from build123d import *

# Parameters (mm, degrees)
SKETCH1_R           = 4.9022
SKETCH1_W           = 40
SKETCH1_H           = 2.6
SKETCH1_W_2         = 80
BOSS_EXTRUDE4_DEPTH = 10


with BuildPart() as part:
    # Sketch1 → Boss-Extrude4 (new body)
    with BuildSketch(Plane(origin=(0, 0, 0), x_dir=(1, 0, 0), z_dir=(0, 1, 0))):
        Polygon((-60.000001624, 254.034119381), (60.000003913, 254.034119381), (250.000001144, -75.055535655), (189.999998376, -178.978582511), (-190.000001624, -178.978582511), (-250.000001624, -75.055534057), align=None)
        with Locations(Location((-200.000000812, -115.470053369, 0), (0, 0, 270))):
            Circle(SKETCH1_R, mode=Mode.SUBTRACT)
        with Locations(Location((199.99999988, -115.470053769, 0), (0, 0, 270))):
            Circle(SKETCH1_R, mode=Mode.SUBTRACT)
        with Locations(Location((5.72e-07, 230.940108145, 0), (0, 0, 270))):
            Circle(SKETCH1_R, mode=Mode.SUBTRACT)
        Polygon((-191.125833025, -87.252540378), (-188.874166975, -85.952540378), (-168.874166975, -120.59355653), (-171.125833025, -121.89355653), align=None, mode=Mode.SUBTRACT)
        with Locations((0, 207.846096908)):
            Rectangle(SKETCH1_W, SKETCH1_H, mode=Mode.SUBTRACT)
        Polygon((188.874166975, -85.952540378), (191.125833025, -87.252540378), (171.125833025, -121.89355653), (168.874166975, -120.59355653), align=None, mode=Mode.SUBTRACT)
        Polygon((148.874166975, -16.670508076), (151.125833025, -17.970508076), (131.125833025, -52.611524227), (128.874166975, -51.311524227), align=None, mode=Mode.SUBTRACT)
        Polygon((-51.125833025, 52.611524227), (-48.874166975, 51.311524227), (-68.874166975, 16.670508076), (-71.125833025, 17.970508076), align=None, mode=Mode.SUBTRACT)
        Polygon((-11.125833025, 121.89355653), (-8.874166975, 120.59355653), (-28.874166975, 85.952540378), (-31.125833025, 87.252540378), align=None, mode=Mode.SUBTRACT)
        Polygon((28.874166975, 52.611524227), (31.125833025, 51.311524227), (11.125833025, 16.670508076), (8.874166975, 17.970508076), align=None, mode=Mode.SUBTRACT)
        Polygon((-61.125833025, 173.855080757), (-58.874166975, 172.555080757), (-98.874166975, 103.273048454), (-101.125833025, 104.573048454), align=None, mode=Mode.SUBTRACT)
        Polygon((-141.125833025, 35.291016151), (-138.874166975, 33.991016151), (-178.874166975, -35.291016151), (-181.125833025, -33.991016151), align=None, mode=Mode.SUBTRACT)
        with Locations((40, 138.564064606)):
            Rectangle(SKETCH1_W, SKETCH1_H, mode=Mode.SUBTRACT)
        with Locations((80, -69.282032303)):
            Rectangle(SKETCH1_W, SKETCH1_H, mode=Mode.SUBTRACT)
        with Locations((-80, -138.564064606)):
            Rectangle(SKETCH1_W_2, SKETCH1_H, mode=Mode.SUBTRACT)
        with Locations((80, -138.564064606)):
            Rectangle(SKETCH1_W_2, SKETCH1_H, mode=Mode.SUBTRACT)
        Polygon((-111.125833025, -87.252540378), (-108.874166975, -85.952540378), (-88.874166975, -120.59355653), (-91.125833025, -121.89355653), align=None, mode=Mode.SUBTRACT)
        Polygon((-71.125833025, -17.970508076), (-68.874166975, -16.670508076), (-48.874166975, -51.311524227), (-51.125833025, -52.611524227), align=None, mode=Mode.SUBTRACT)
        Polygon((8.874166975, -17.970508076), (11.125833025, -16.670508076), (31.125833025, -51.311524227), (28.874166975, -52.611524227), align=None, mode=Mode.SUBTRACT)
        Polygon((48.874166975, 51.311524227), (51.125833025, 52.611524227), (71.125833025, 17.970508076), (68.874166975, 16.670508076), align=None, mode=Mode.SUBTRACT)
        Polygon((58.863601684, 172.573380377), (61.115267734, 173.873380377), (101.115267734, 104.591348074), (98.863601684, 103.291348074), align=None, mode=Mode.SUBTRACT)
        Polygon((138.874166975, 33.991016151), (141.125833025, 35.291016151), (181.125833025, -33.991016151), (178.874166975, -35.291016151), align=None, mode=Mode.SUBTRACT)
    extrude(amount=BOSS_EXTRUDE4_DEPTH)


solid = part.part
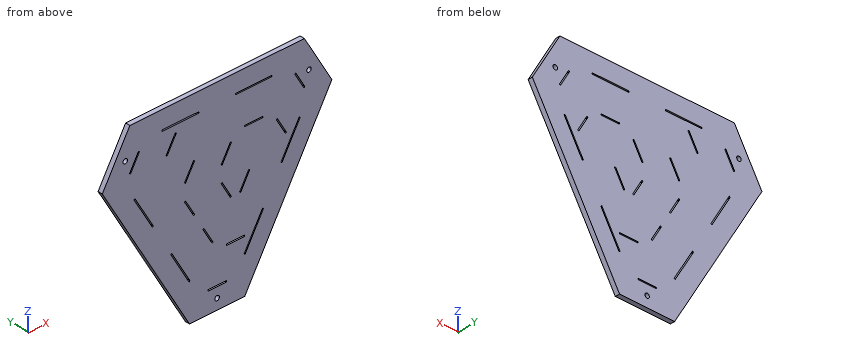
Check sheet for the modelled part. Datum: model origin and axes. Units: mm. Round coordinates to 2 decimals unless told otherwise and drop trailing zeros. Write each loop counter-clockwise with the first axis right and the second up, starting at its lowest first coordinate (ties: lowest second). Pieces come first, ordered by that corner, then holes. Notation, with made-up numbers: (12, 31) - (63, 31) arc R33 cw to (63, 70) - close; hole circle Ø7 at (46.5, 70). An arc over 180 degrees is marked (long way). Return JSON: item names as keys, results as strings.
Q1. Cross-section at B-B (y = 4). Give the number of separate pieces and of enclosed holes in the cut face, then the cut area to 3 significant figures.
Returned:
{"separate pieces": "1", "enclosed holes": "22", "area": "145,000 mm²"}
Q2. Depth check by flat-ended pin: P1, Ø3, axis at y = 4, z = 139, coming from the -X side; P2, Ø12.5, axis at x = -200, z = 115.47, coming from the +Y side; P3, Ø5, axis at y = 5.5, z = -10, coming from the +X side; P4, Ø3, axis at y = 6.5, z = -207.5, coming from the -X side. Enter the tip coordinate at first touch or a pass-through.
Returned:
{"P1": "stops at x = -213.95", "P2": "stops at y = 10", "P3": "stops at x = 202.34", "P4": "stops at x = -87.73"}
Q3. Cross-section at C-C (z = -71). Record the boundary of the cut face in (x, y).
Returned:
{"outline": "(-165.67, 0) - (165.67, 0) - (165.67, 10) - (-165.67, 10) - close"}
Q4. Cross-section at A-A (z = -129). Record the boundary of the cut face in (x, y).
Returned:
{"outline": "(-132.19, 0) - (-87.02, 0) - (-87.02, 10) - (-132.19, 10) - close; (-84.02, 0) - (84.02, 0) - (84.02, 10) - (-84.02, 10) - close; (87.02, 0) - (132.19, 0) - (132.19, 10) - (87.02, 10) - close"}
Q5. Scan lines: L1, parallel to X at y = 4, z = -24; L2, parallel to X at y = 6, z = 42.5; L3, parallel to X at y = 7.25, z = 119.5. Record each from-to range of solid material in increasing order. Write a range as from..to.
Returned:
{"L1": "x = -192.81..-147.64, -144.64..-67.64, -64.64..12.36, 15.36..64.64, 67.64..144.64, 147.64..192.81", "L2": "x = -231.2..-56.96, -53.96..23.04, 26.04..133.96, 136.96..231.2", "L3": "x = -224.34..-202.79, -197.21..-172.51, -169.51..-92.51, -89.51..169.51, 172.51..197.21, 202.79..224.34"}
